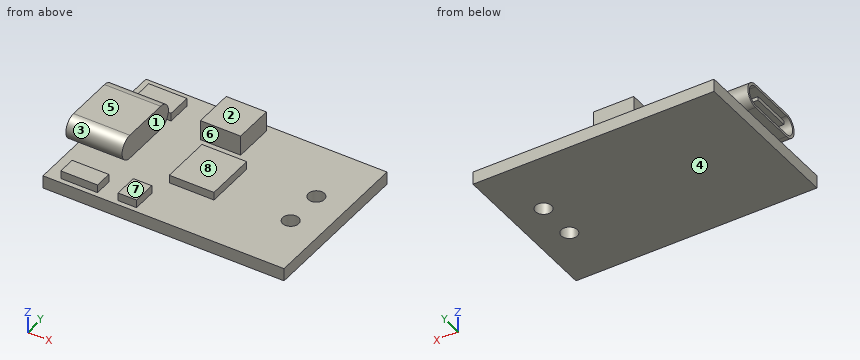
from build123d import *

# Parameters (mm, degrees)
SKICA1_W                     = 30
SKICA1_H                     = 20
P_IDAT_VYSUNUT_M1_DEPTH      = 1.6
SKICA2_W                     = 5
SKICA2_H                     = 5
P_IDAT_VYSUNUT_M2_DEPTH      = 2.5
SKICA3_W                     = 5.560208965
SKICA3_H                     = 6.363350261
SKICA3_W_2                   = 2.285863686
SKICA3_H_2                   = 2.965444781
SKICA3_W_3                   = 4.571727371
SKICA3_H_3                   = 2.193193536
SKICA3_W_4                   = 4.75706767
SKICA3_H_4                   = 3.089004981
P_IDAT_VYSUNUT_M3_DEPTH      = 1
SKICA4_R                     = 1
ODEBRAT_VYSUNUT_M1_DEPTH     = 11
P_IDAT_VYSUNUT_M4_DEPTH      = 1
P_IDAT_VYSUNUT_M4_DEPTH_BACK = 6
SKICA6_W                     = 0.458188224
SKICA6_H                     = 5.040283318
ODEBRAT_VYSUNUT_M2_DEPTH     = 6


with BuildPart() as part:
    # Skica1 → Přidat vysunutím1 (new body)
    with BuildSketch(Plane.XY):
        with Locations((15, 10)):
            Rectangle(SKICA1_W, SKICA1_H)
    extrude(amount=P_IDAT_VYSUNUT_M1_DEPTH)

    # Skica2 → Přidat vysunutím2 (add)
    with BuildSketch(Plane.XY.offset(1.6)):
        with Locations((13, 16.7)):
            Rectangle(SKICA2_W, SKICA2_H)
    extrude(amount=P_IDAT_VYSUNUT_M2_DEPTH)

    # Skica3 → Přidat vysunutím3 (add)
    with BuildSketch(Plane.XY.offset(1.6)):
        with Locations((14.582984328, 9.289528855)):
            Rectangle(SKICA3_W, SKICA3_H)
        with Locations((10.103927106, 2.092147249)):
            Rectangle(SKICA3_W_2, SKICA3_H_2)
        with Locations((4.111257444, 1.706021627)):
            Rectangle(SKICA3_W_3, SKICA3_H_3)
        with Locations((3.771466895, 16.826701007)):
            Rectangle(SKICA3_W_4, SKICA3_H_4)
    extrude(amount=P_IDAT_VYSUNUT_M3_DEPTH)

    # Skica4 → Odebrat vysunutím1 (cut)
    with BuildSketch(Plane.XY.offset(1.6)):
        with Locations((26.071400283, 12.424560679)):
            Circle(SKICA4_R)
        with Locations((26.071400283, 7.424560679)):
            Circle(SKICA4_R)
    extrude(amount=-ODEBRAT_VYSUNUT_M1_DEPTH, mode=Mode.SUBTRACT)

    # Skica5 → Přidat vysunutím4 (add, two sides: drawn at the far end of the back side and taken through both)
    with BuildSketch(Plane.ZY.offset(-P_IDAT_VYSUNUT_M4_DEPTH_BACK)):
        with BuildLine():
            Line((4.6, 13.5), (4.6, 7.5))
            ThreePointArc((4.6, 7.5), (3.1, 6), (1.6, 7.5))
            Line((1.6, 7.5), (1.6, 13.5))
            ThreePointArc((1.6, 13.5), (3.1, 15), (4.6, 13.5))
        make_face()
    extrude(amount=P_IDAT_VYSUNUT_M4_DEPTH + P_IDAT_VYSUNUT_M4_DEPTH_BACK)

    # Skica6 → Odebrat vysunutím2 (cut)
    with BuildSketch(Plane.ZY.offset(1)):
        with BuildLine():
            Line((1.9, 13.5), (1.9, 7.5))
            ThreePointArc((1.9, 7.5), (3.1, 6.3), (4.3, 7.5))
            Line((4.3, 7.5), (4.3, 13.5))
            ThreePointArc((4.3, 13.5), (3.1, 14.7), (1.9, 13.5))
        make_face()
        with Locations((3.1, 10.5)):
            Rectangle(SKICA6_W, SKICA6_H, mode=Mode.SUBTRACT)
    extrude(amount=-ODEBRAT_VYSUNUT_M2_DEPTH, mode=Mode.SUBTRACT)


solid = part.part
Geometry check sheet. Reference: the model listing, model coordinates, mm. Face numbers are marked on the shaded views. A direction names the side the tool comes from. Give positions to 0.01 mm unless a question says otherwise; leave off trailing zeros. Order: outer loops, then holes, each group sorted by start corner. A loop starts at its lowest first (then second) coordinate and runs counter-clockwise, first axis right, second up.
1. Draft check along Z on the marked faces 1, 2, 3 and 4. Enter one of: pulls with the +Z half, pulls with the -Z half, needs draft (parallel to the pull), parting line crosses it, or undercut.
Completed:
face 1: needs draft
face 2: pulls with the +Z half
face 3: undercut
face 4: pulls with the -Z half
2. Scan lines: line 1 (Y direction, x = 1, z = 3.15); line 2 (X direction, y = 1.5, z = 2.1); line 3 (X direction, y = 14.75, z = 2.9). Record each from-to range of solid material in increasing order.
Completed:
line 1: y = 6 to 6.3, 7.98 to 13.02, 14.7 to 15
line 2: x = 1.83 to 6.4, 8.96 to 11.25
line 3: x = -1 to 6, 10.5 to 15.5
3. Access from +Z, -Z, +X, -X, +Y, -Y to the whole of each face (thin tool, end or side, straight path). Record for the marked faces 5, 6, 7 and 8.
Completed:
face 5: +Z, +X, -X, +Y, -Y
face 6: +Z, +X
face 7: +Z, +X, -X, -Y
face 8: +Z, +X, -Y
4. Depth check by flat-ended pin: pin 1 (6 mm diameter, centred on x = 14, y = 9, fed in from +Z); pin 2 (0.5 mm diameter, centred on y = 16, z = 2, fed in from +X); pin 3 (0.8 mm diameter, centred on y = 9.5, z = 2.5, fed in from +X). Enter the tip coordinate at first touch or a pass-through.
Completed:
pin 1: stops at z = 2.6
pin 2: stops at x = 15.5
pin 3: stops at x = 17.36
5. Sectioned sample at A-A (x = 2.5). Record the boundary of the cut face in (y, z), then the cut area to 3 significant figures.
Completed:
outline: (0, 0) - (20, 0) - (20, 1.6) - (18.37, 1.6) - (18.37, 2.6) - (15.28, 2.6) - (15.28, 1.6) - (13.5, 1.6) arc R1.5 ccw to (13.5, 4.6) - (7.5, 4.6) arc R1.5 ccw to (7.5, 1.6) - (2.8, 1.6) - (2.8, 2.6) - (0.61, 2.6) - (0.61, 1.6) - (0, 1.6) - close; (7.98, 2.87) - (13.02, 2.87) - (13.02, 3.33) - (7.98, 3.33) - close; hole (7.5, 1.9) - (13.5, 1.9) arc R1.2 ccw to (13.5, 4.3) - (7.5, 4.3) arc R1.2 ccw to start
area: 45.7 mm2
6. Sectioned sample at D-D (x = 13). Record the boundary of the cut face in (y, z), then the cut area to 3 significant figures.
Completed:
outline: (0, 0) - (20, 0) - (20, 1.6) - (19.2, 1.6) - (19.2, 4.1) - (14.2, 4.1) - (14.2, 1.6) - (12.47, 1.6) - (12.47, 2.6) - (6.11, 2.6) - (6.11, 1.6) - (0, 1.6) - close
area: 50.9 mm2
7. Sectioned sample at B-B (z = 2.2). Record the boundary of the cut face in (x, y).
Completed:
outline: (-1, 6.3) - (6, 6.3) - (6, 14.7) - (-1, 14.7) - (-1, 14.29) - (5, 14.29) - (5, 6.71) - (-1, 6.71) - close; (1.39, 15.28) - (6.15, 15.28) - (6.15, 18.37) - (1.39, 18.37) - close; (1.83, 0.61) - (6.4, 0.61) - (6.4, 2.8) - (1.83, 2.8) - close; (8.96, 0.61) - (11.25, 0.61) - (11.25, 3.57) - (8.96, 3.57) - close; (10.5, 14.2) - (15.5, 14.2) - (15.5, 19.2) - (10.5, 19.2) - close; (11.8, 6.11) - (17.36, 6.11) - (17.36, 12.47) - (11.8, 12.47) - close
8. Sectioned sample at C-C (y = 18). Record the boundary of the cut face in (x, z).
Completed:
outline: (0, 0) - (30, 0) - (30, 1.6) - (15.5, 1.6) - (15.5, 4.1) - (10.5, 4.1) - (10.5, 1.6) - (6.15, 1.6) - (6.15, 2.6) - (1.39, 2.6) - (1.39, 1.6) - (0, 1.6) - close
